```python
from build123d import *

# Parameters (mm, degrees)
F0_W     = 200
F0_H     = 100
F1_DEPTH = 110
F2_W     = 200
F2_H     = 100
F3_DEPTH = 25
F5_DEPTH = 100


with BuildPart() as f1:
    # F0 (on Front) → F1 (new body)
    with BuildSketch(Plane.XZ):
        Rectangle(F0_W, F0_H)
        Polygon((-60, -24.5), (-72.5, 24.5), (72.5, 24.5), (60, -24.5), align=None, mode=Mode.SUBTRACT)
    extrude(amount=-F1_DEPTH)

    # F2 (on face) → F3 (join)
    with BuildSketch(Plane(origin=(0, 110, 0), x_dir=(-1, 0, 0), z_dir=(0, 1, 0))):
        Rectangle(F2_W, F2_H)
    extrude(amount=F3_DEPTH)

    # F4 (on Right) → F5 (join, symmetric)
    with BuildSketch(Plane.YZ):
        with BuildLine():
            Line((-75, -50), (0, -50))
            Line((0, -50), (0, -19.5))
            add(Edge.make_bspline(
                [(0, -19.5), (-5.83801, -19.088345), (-16.211687, -12.465747), (-20, -9.5)],
                knots=[0, 0, 0, 0, 22.36068, 22.36068, 22.36068, 22.36068], degree=3))
            Line((-20, -9.5), (-75, -9.5))
            Line((-75, -9.5), (-75, -50))
        make_face()
    extrude(amount=F5_DEPTH, both=True)


solid = f1.part
```
Input: part model. Units: mm. Frame: model coordinates. A direction names the side the tool comes from. Coordinates: 2 decimals unless noted, no trailing zeros. Order: outer loops, then holes, each group sorted by start corner. A loop starts at its lowest first (then second) coordinate and runs counter-clockwise, first axis right, second up. Notation, with made-up numbers: (-7, -23) - (20, -23) arc R35 cw to (20, 13) - close; hole circle Ø8 at (-9, 88). An arc over 180 degrees is marked (long way). Return JSON: item names as keys, results as strings.
Q1. Access query for faces 4 (the flat face through (100, 52, 1)), 5 (the flat face through (-66.162, 54.23, -0.343)), 6 (the flat face through (-1, 54, 24.5)). Directions: +Z, -Z, +X, -X, +Y, -Y. A direction counts if a zero-diameter tool reaches every point of the face in a straight line with its end or side. Return the directions, or none.
The answers:
{"face 4": "+Z, -Z, +X, +Y, -Y", "face 5": "none", "face 6": "-Y"}
Q2. Cut plane B-B (z = 32). Return loops of the section in (x, y), then the cut area to 3 significant figures.
The answers:
{"outline": "(-100, 0) - (100, 0) - (100, 135) - (-100, 135) - close", "area": "27,000 mm2"}
Q3. Ray query, probe 1 along Z at (x, y) = (52.5, 5); probe 2 along Y at (x, z) = (16.5, 15.5); probe 3 along Y at (x, z) = (10, 37). Return the intervals inside material, ascending.
The answers:
{"probe 1": "z = -50 to -24.5, 24.5 to 50", "probe 2": "y = 110 to 135", "probe 3": "y = 0 to 135"}
Q4. Cut plane A-A (y = 75.5). Return loops of the section in (x, z).
The answers:
{"outline": "(-100, -50) - (100, -50) - (100, 50) - (-100, 50) - close; hole (-72.5, 24.5) - (-60, -24.5) - (60, -24.5) - (72.5, 24.5) - close"}
Q5. Draft query along Z for faces 1 (the flat face through (1, 54, -24.5)), 2 (the flat face through (1, 135, 1)), 3 (the flat face through (1, -47, -9.5)). Return one class per face: +Z half, -Z half, draft (parallel to the pull), parting line (faces both ways), or undercut.
The answers:
{"face 1": "undercut", "face 2": "draft", "face 3": "+Z half"}
